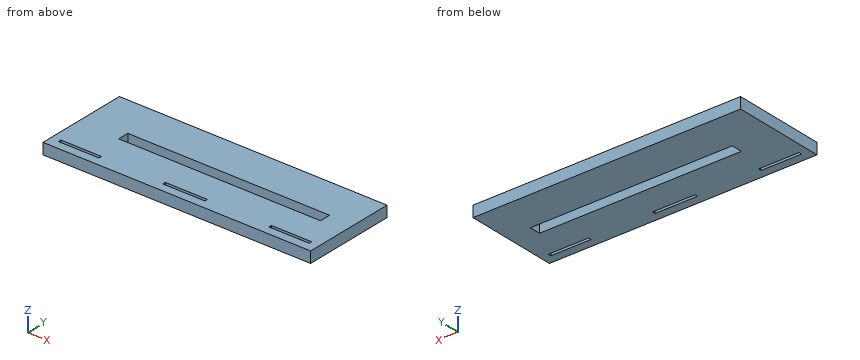
Autodesk Inventor part; units mm, degrees
ref_plane "Work Plane1" through (0, 23, 0) normal (0, 1, 0) x (1, 0, 0)
ref_plane "Work Plane2" through (66.3, 0, 0) normal (1, 0, 0) x (0, 0, -1)
ref_plane "YZ Plane" through (0, 0, 0) normal (1, 0, 0) x (0, 1, 0)
sketch "Sketch1" plane through (0, 0, 0) normal (0, 0, 1) x (1, 0, 0)
  line L0 (0, 0) -> (132.6, 0)
  line L1 (132.6, 0) -> (132.6, 46)
  line L2 (132.6, 46) -> (0, 46)
  line L3 (0, 46) -> (0, 0)
  line L4 (66.3, 46) -> (66.3, 0) construction
  line L5 (55.85, 4.25) -> (76.75, 4.25)
  line L6 (76.75, 4.25) -> (76.75, 5.75)
  line L7 (76.75, 5.75) -> (55.85, 5.75)
  line L8 (55.85, 5.75) -> (55.85, 4.25)
  line L9 (55.85, 4.25) -> (76.75, 5.75) construction
  line L10 (76.75, 4.25) -> (55.85, 5.75) construction
  line L11 (4.2, 5.75) -> (24.2, 5.75)
  line L12 (24.2, 5.75) -> (24.2, 4.25)
  line L13 (24.2, 4.25) -> (4.2, 4.25)
  line L14 (4.2, 4.25) -> (4.2, 5.75)
  line L15 (4.2, 5.75) -> (24.2, 4.25) construction
  line L16 (24.2, 5.75) -> (4.2, 4.25) construction
  line L17 (108.4, 4.25) -> (128.4, 4.25)
  line L18 (128.4, 4.25) -> (128.4, 5.75)
  line L19 (128.4, 5.75) -> (108.4, 5.75)
  line L20 (108.4, 5.75) -> (108.4, 4.25)
  line L21 (108.4, 4.25) -> (128.4, 5.75) construction
  line L22 (128.4, 4.25) -> (108.4, 5.75) construction
  line L23 (14.2, 5) -> (118.4, 5) construction
  point P0 (66.3, 5)
  point P1 (66.3, 5)
  dimension "d0" = 132.6
  dimension "d1" = 46
  dimension "d2" = 1.5
  dimension "d3" = 20.9
  dimension "d4" = 1.5
  dimension "d5" = 20
  dimension "d7" = 20
  dimension "d8" = 1.5
  dimension "d17" = 5
  dimension "d18" = 52.1
extrude "Extrusion1" add sketch "Sketch1" along normal blind 5.5
ref_plane "Work Plane1" through (0, 23, 0) normal (0, 1, 0) x (1, 0, 0)
ref_plane "Work Plane2" through (66.3, 0, 0) normal (1, 0, 0) x (0, 0, -1)
ref_plane "Work Plane3" through (4.2, 5, 0) normal (0, 1, 0) x (1, 0, 0)
sketch "Sketch3" plane through (0, 0, 5.5) normal (0, 0, 1) x (1, 0, 0)
  line L0 (20.6246, 26) -> (120.6246, 26)
  line L1 (120.6246, 26) -> (120.6246, 20.5)
  line L2 (120.6246, 20.5) -> (20.6246, 20.5)
  line L3 (20.6246, 20.5) -> (20.6246, 26)
  line L4 (132.6, 46) -> (0, 46)
  point P0 (0, 0)
  dimension "d19" = 100
  dimension "d20" = 5.5
  dimension "d21" = 20
extrude "Extrusion2" cut sketch "Sketch3" against normal blind 5.5
equation "\"d3\" = lrmid + toler"
equation "\"d4\" = d2"
equation "\"d5\" = lrlr + toler"
equation "\"d7\" = d5"
equation "\"d8\" = d2"
equation "\"thick\" = 0.5"
equation "\"lrlr\" = 19"
equation "\"lrmid\" = 19.9"
equation "\"lrdepth\" = 3.3"
equation "\"mlr\" = 16.6"
equation "\"mmid\" = 24.7"
equation "\"mdepth\" = 4.5"
equation "\"lrltotal\" = 126.6"
equation "\"mltotal\" = 126.6"
equation "\"lrbetween\" = 52.1"
equation "\"mbetween\" = 49.5"
equation "\"toler\" = 1"
equation "\"stuckw\" = 6"
equation "\"tight\" = 0.08"
equation "\"sidewallL\" = 132.6"
equation "\"heaterH\" = 117.3"
equation "\"stickL\" = 3.5"
equation "\"wireH\" = 25"
properties part number "lr_bottom"
For this review, take the finished solid that the model builds, in its own axes (mm). Coordinates: 2 decimals unless noted, no trailing zeros. Loops run counter-clockwise (first coordinate to the right, second up) from the corner with the lowest first, then second, coordinate; pieces in that order, holes last. Notation, with made-up numbers: (-8.75, 26.25) - (42.25, 26.25) arc R19 ccw to (42.25, 46.25) - close; hole circle Ø4 at (69.25, 43.25). An arc over 180 degrees is marked (long way). Return JSON: item names as keys, results as strings.
Item 1: Take a section at C-C (z = 2.8). Give the boundary of the cut face in (x, y), then the cut area to 3 significant figures.
Determined:
{"outline": "(0, 0) - (132.6, 0) - (132.6, 46) - (0, 46) - close; hole (4.2, 4.25) - (24.2, 4.25) - (24.2, 5.75) - (4.2, 5.75) - close; hole (20.62, 20.5) - (120.62, 20.5) - (120.62, 26) - (20.62, 26) - close; hole (55.85, 4.25) - (76.75, 4.25) - (76.75, 5.75) - (55.85, 5.75) - close; hole (108.4, 4.25) - (128.4, 4.25) - (128.4, 5.75) - (108.4, 5.75) - close", "area": "5,460 mm2"}
Item 2: Take a section at A-A (x = 18). Give the boundary of the cut face in (y, z).
Determined:
{"outline": "(0, 0) - (4.25, 0) - (4.25, 5.5) - (0, 5.5) - close; (5.75, 0) - (46, 0) - (46, 5.5) - (5.75, 5.5) - close"}
Item 3: Take a section at B-B (x = 57.5). Give the boundary of the cut face in (y, z), then the cut area to 4 significant figures.
Determined:
{"outline": "(0, 0) - (4.25, 0) - (4.25, 5.5) - (0, 5.5) - close; (5.75, 0) - (20.5, 0) - (20.5, 5.5) - (5.75, 5.5) - close; (26, 0) - (46, 0) - (46, 5.5) - (26, 5.5) - close", "area": "214.5 mm2"}
Item 4: For line 1 (Y direction, x = 59, z = 0.8); line 2 (Y direction, x = 11.5, z = 3.55); line 3 (Y direction, x = 24.5, z = 4.2), list the stretches that pass through material, from the lowest coordinate up.
Determined:
{"line 1": "y = 0 to 4.25, 5.75 to 20.5, 26 to 46", "line 2": "y = 0 to 4.25, 5.75 to 46", "line 3": "y = 0 to 20.5, 26 to 46"}
